from build123d import *

# Parameters (mm, degrees)
BOSS_EXTRUDE1_DEPTH = 3
SKETCH4_W           = 40
SKETCH4_H           = 3
BOSS_EXTRUDE2_DEPTH = 10
FILLET1_R           = 2
FILLET2_R           = 2
SKETCH5_R           = 1.5
CUT_EXTRUDE1_DEPTH  = 27.787357167
SKETCH6_R           = 3.5
BOSS_EXTRUDE3_DEPTH = 16
FILLET3_R           = 0.5
SKETCH7_W           = 10
SKETCH7_H           = 8.75
BOSS_EXTRUDE4_DEPTH = 1.5
FILLET4_R           = 1


with BuildPart() as part:
    # Sketch3 → Boss-Extrude1 (new body)
    with BuildSketch(Plane.XY):
        with BuildLine():
            Line((-0.1, -6), (-10.1, -6))
            ThreePointArc((-10.1, -6), (-10.708761429, -5.79335334), (-11.065925826, -5.258819045))
            Line((-11.065925826, -5.258819045), (-13.886481515, 5.26763809))
            ThreePointArc((-13.886481515, 5.26763809), (-14.600810309, 6.336706681), (-15.818333167, 6.75))
            Line((-15.818333167, 6.75), (-19, 6.75))
            ThreePointArc((-19, 6.75), (-19.707106781, 7.042893219), (-20, 7.75))
            Line((-20, 7.75), (-20, 11.75))
            Line((-20, 11.75), (20, 11.75))
            Line((20, 11.75), (20, 7.75))
            ThreePointArc((20, 7.75), (19.707106781, 7.042893219), (19, 6.75))
            Line((19, 6.75), (5.618333167, 6.75))
            ThreePointArc((5.618333167, 6.75), (4.400810309, 6.336706681), (3.686481515, 5.26763809))
            Line((3.686481515, 5.26763809), (0.865925826, -5.258819045))
            ThreePointArc((0.865925826, -5.258819045), (0.508761429, -5.79335334), (-0.1, -6))
        make_face()
    extrude(amount=BOSS_EXTRUDE1_DEPTH)

    # Sketch4 → Boss-Extrude2 (add)
    with BuildSketch(Plane(origin=(0, 0, 0), x_dir=(-1, 0, 0), z_dir=(0, 0, -1))):
        with Locations((0, 10.25)):
            Rectangle(SKETCH4_W, SKETCH4_H)
    extrude(amount=BOSS_EXTRUDE2_DEPTH)

    # Fillet1
    fillet1_edges = [part.edges().sort_by_distance(p)[0] for p in [
        (0, 8.75, 0),
    ]]
    fillet(fillet1_edges, radius=FILLET1_R - 0.0001)  # a hair under: the kernel refuses the full size

    # Fillet2
    fillet2_edges = [part.edges().sort_by_distance(p)[0] for p in [
        (20, 10.25, -10),
        (-20, 10.25, -10),
    ]]
    fillet(fillet2_edges, radius=FILLET2_R)

    # Sketch5 → Cut-Extrude1 (cut, through all)
    with BuildSketch(Plane.XZ.offset(-8.75)):
        with Locations(Location((-16, -6, 0), (0, 0, 270))):
            Circle(SKETCH5_R)
    cut_extrude1 = extrude(amount=-CUT_EXTRUDE1_DEPTH, mode=Mode.SUBTRACT)

    # Mirror1: Cut-Extrude1 across plane
    add(cut_extrude1.mirror(Plane(origin=(0, 0, 0), x_dir=(0, 0, 1), z_dir=(1, 0, 0))), mode=Mode.SUBTRACT)

    # Sketch6 → Boss-Extrude3 (add)
    with BuildSketch(Plane(origin=(0, 0, 0), x_dir=(-1, 0, 0), z_dir=(0, 0, -1))):
        with Locations((5.1, 0)):
            Circle(SKETCH6_R)
    extrude(amount=BOSS_EXTRUDE3_DEPTH)

    # Fillet3
    fillet3_edges = [part.edges().sort_by_distance(p)[0] for p in [
        (-1.6, 0, -16),
    ]]
    fillet(fillet3_edges, radius=FILLET3_R)

    # Sketch7 → Boss-Extrude4 (add, symmetric)
    with BuildSketch(Plane(origin=(-5.1, 0, 0), x_dir=(0, 0, -1), z_dir=(1, 0, 0))):
        with Locations((5, 4.375)):
            Rectangle(SKETCH7_W, SKETCH7_H)
    extrude(amount=BOSS_EXTRUDE4_DEPTH, both=True)

    # Fillet4
    fillet4_edges = [part.edges().sort_by_distance(p)[0] for p in [
        (-3.6, 8.164242852, -0.585757148),
        (-6.6, 4.95618883, 0),
        (-6.6, 8.164242852, -0.585757148),
        (-6.6, 8.75, -5.99995),
        (-3.6, 8.75, -5.99995),
        (-3.6, 4.95618883, 0),
        (-6.6, 3.16227766, -5),
        (-5.1, 3.5, -10),
        (-3.6, 3.16227766, -5),
    ]]
    fillet(fillet4_edges, radius=FILLET4_R)


solid = part.part
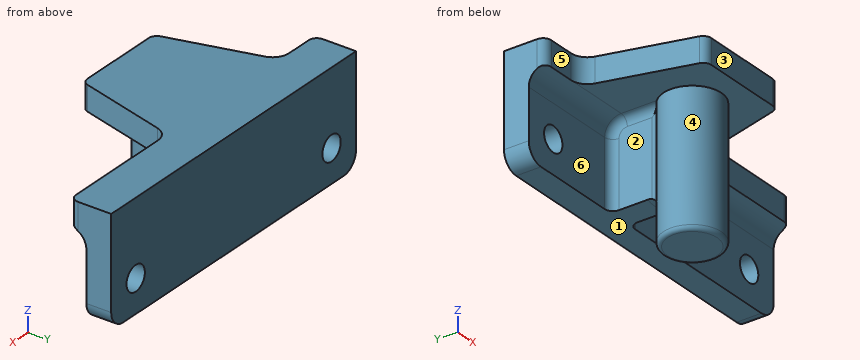
For this review, take the finished solid that the model builds, in its own axes (mm). Face numbers are marked on the shaded views. A direction names the side the tool comes from. Give positions to 0.01 mm unless a question says otherwise; leave off trailing zeros. Loops run counter-clockwise (first coordinate to the right, second up) from the corner with the lowest first, then second, coordinate; pieces in that order, holes last. Notation, with made-up numbers: (-16.5, -34.75) - (-5.5, -34.75) arc R28 cw to (-5.5, 0.25) - close; hole circle Ø5 at (24.5, -22). An arc over 180 degrees is marked (long way). Write each question's results on one line, items separated by ' | '.
(1) Take a section at C-C (x = -5.1). Give the boundary of the cut face in (y, z), then the cut area to 3 significant figures.
Conclusion:
outline: (-6, 0) - (-3.5, 0) - (-3.5, -15.5) arc R0.5 ccw to (-3, -16) - (3, -16) arc R0.5 ccw to (3.5, -15.5) - (3.5, -11) arc R1 cw to (4.5, -10) - (11.75, -10) - (11.75, 3) - (-6, 3) - close | area: 248 mm^2
(2) Take a section at A-A (y = 10). Give the boundary of the cut face in (x, z), then the cut area to 3 significant figures.
Conclusion:
outline: (-20, -8) arc R2 ccw to (-18, -10) - (18, -10) arc R2 ccw to (20, -8) - (20, 3) - (-20, 3) - close; hole circle Ø3 at (-16, -6); hole circle Ø3 at (16, -6) | area: 504 mm^2
(3) Take a section at D-D (z = -7). Give the boundary of the cut face in (x, y), then the cut area to 3 significant figures.
Conclusion:
outline: (-20, 8.75) - (-17.12, 8.75) - (-17.12, 11.75) - (-20, 11.75) - close; (-14.88, 8.75) - (-7.6, 8.75) arc R1 cw to (-6.6, 7.75) - (-6.6, 3.74) arc R1 cw to (-7.04, 2.91) arc R3.5 ccw (long way) to (-3.16, 2.91) arc R1 cw to (-3.6, 3.74) - (-3.6, 7.75) arc R1 cw to (-2.6, 8.75) - (14.88, 8.75) - (14.88, 11.75) - (-14.88, 11.75) - close; (17.12, 8.75) - (20, 8.75) - (20, 11.75) - (17.12, 11.75) - close | area: 162 mm^2
(4) For pin 1 Ø4 at (x, y) = (-2.5, 6) entering from -Z; pin 2 Ø5 at (x, y) = (10, 6) entering from +Z; pin 3 Ø3 at (y, z) = (5.5, -6) entering from +X; pin 4 Ø4.5 at (y, z) = (6, -7) entering from -X, all flat-tipped, find the tip position at first contact; note any pin that passes through.
Conclusion:
pin 1: z = -10 | pin 2: z = 3 | pin 3: x = -3.6 | pin 4: x = -6.73
(5) Draft analysis for pull direction Y (two halves, no side actions). For the marked faces 1, 2 and 3, state which applies: +Y half, -Y half, draft (parallel to the pull), parting line (faces both ways), or undercut.
Conclusion:
face 1: draft | face 2: undercut | face 3: -Y half
(6) For line 1 along X through (y, z) = (11.15, -6); line 2 along Z through (x, y) = (9.5, 9.25); line 3 along X through (y, z) = (-0.25, -11), list the stretches that pass through material, from the lowest coordinate up.
Conclusion:
line 1: -20 to -17.5, -14.5 to 14.5, 17.5 to 20 | line 2: -10 to 3 | line 3: -8.59 to -1.61
(7) For the marked faces 4, 5 and 6, list the 3-axis set-ups (+Z, -Z, +X, -X, +Y, -Y) from which the entire face can be reached by the end or side of a thin tool; tool diameter is ignored.
Conclusion:
face 4: -Z | face 5: +Z, -Z, -X, -Y | face 6: -Z, -X
